Job drawing, mm, ordinate dimensions from the low corner. One solid piece. Coordinates: 2 decimals unless noted, no trailing zeros. Order: outer loops, then holes, each group sorted by start corner. A loop starts at its lowest first (then second) coordinate and runs counter-clockwise, first axis right, second up. Notation, with made-up numbers: (16, -38) - (66, -38) arc R27 ccw to (66, 1) - close; hole circle Ø4 at (23, 82). An arc over 180 degrees is marked (long way). Return JSON: item names as keys, results as strings.
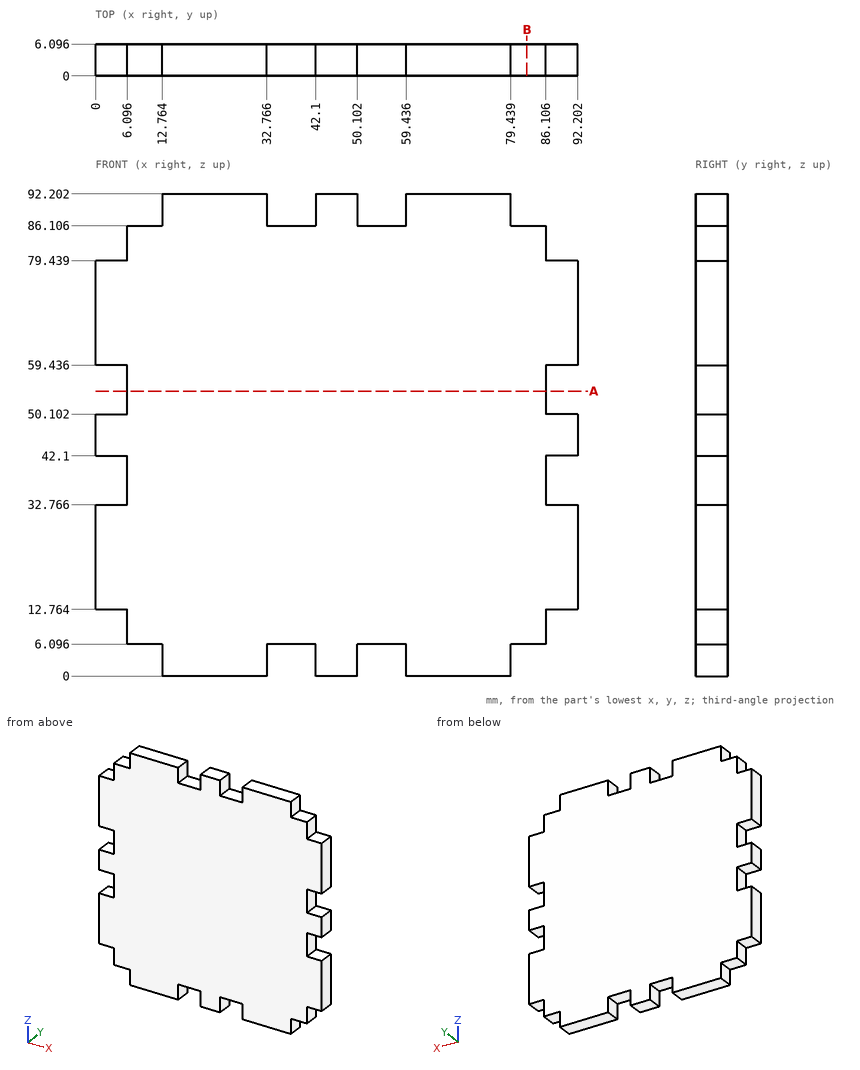
1. Cut at A-A on z = 54.5. Give the cut face in (x, y) (1 decimal), plus the area to 3 significant figures.
Check values:
{"outline": "(6.1, 0) - (86.1, 0) - (86.1, 6.1) - (6.1, 6.1) - close", "area": "488 mm²"}
2. Cut at B-B on x = 82.5. Give the cut face in (y, z) (1 decimal).
Check values:
{"outline": "(0, 6.1) - (6.1, 6.1) - (6.1, 86.1) - (0, 86.1) - close"}
3. Drop flat-ended pins along their axis: pin 1 (1.8 mm diameter, centred on y = 3.5, z = 53.5, fed in from +X); pin 2 (1.8 mm diameter, centred on x = 84, y = 4.5, fed in from -Z); pin 3 (1.8 mm diameter, centred on x = 89.5, y = 2, fed in from +Z); pin 4 (2 mm diameter, centred on y = 2.5, z = 18.5, fed in from -X). Give the stop position or say it passes through.
Check values:
{"pin 1": "x = 86.11", "pin 2": "z = 6.1", "pin 3": "z = 79.44", "pin 4": "x = 0"}
4. Probe L1, parallel to Z at x = 86.5, y = 2.75 (1 decimal); L2, parallel to Z at x = 54, y = 3.25 (1 decimal). List the from-to ranges inside material, lowest first.
Check values:
{"L1": "12.8 to 32.8, 42.1 to 50.1, 59.4 to 79.4", "L2": "6.1 to 86.1"}
